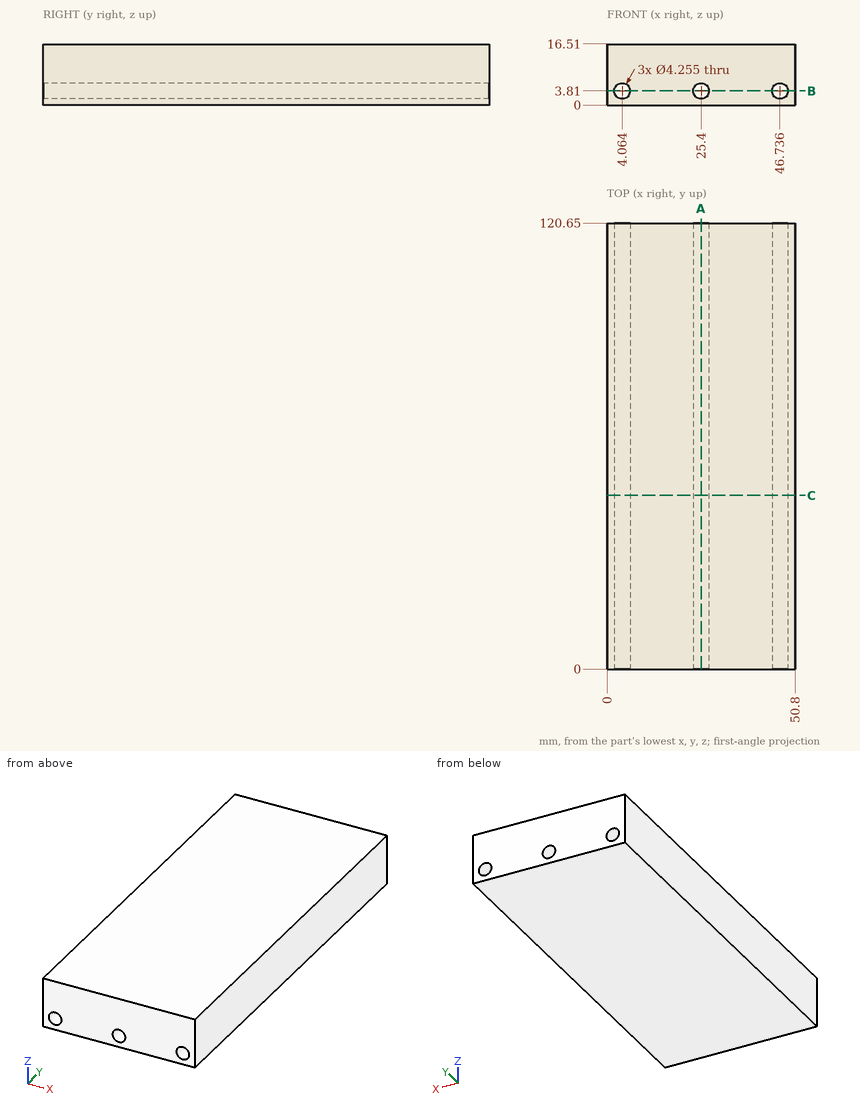
Part print with two shaded views. Sizes in mm from the minimum x, y, z corner. Give positions to 0.01 mm unless a question says otherwise; leave off trailing zeros. Order: outer loops, then holes, each group sorted by start corner. A loop starts at its lowest first (then second) coordinate and runs counter-clockwise, first axis right, second up. Notation, with made-up numbers: M 54.25,16 L 103.25,16 A20 cw 103.25,34 Z; hole C 53.5,14 d6. An arc over 180 degrees is marked long. Write item = value, one per line.
Q1. Cut at B-B, the plane z = 3.81. List the corners of the cut face in (x, y), then the cut area to 3 significant figures.
Derived:
outline = M 0,0 L 1.94,0 L 1.94,120.65 L 0,120.65 Z; M 6.19,0 L 23.27,0 L 23.27,120.65 L 6.19,120.65 Z; M 27.53,0 L 44.61,0 L 44.61,120.65 L 27.53,120.65 Z; M 48.86,0 L 50.8,0 L 50.8,120.65 L 48.86,120.65 Z
area = 4,590 mm2
Q2. Cut at A-A, the plane x = 25.4. List the corners of the cut face in (y, z), then the cut area to 3 significant figures.
Derived:
outline = M 0,0 L 120.65,0 L 120.65,1.68 L 0,1.68 Z; M 0,5.94 L 120.65,5.94 L 120.65,16.51 L 0,16.51 Z
area = 1,480 mm2
Q3. Drill centre lines: line 1 (X direction, y = 79, z = 3.81); line 2 (X direction, y = 38, z = 5.25) (1 decimal); line 3 (Z direction, x = 46, y = 9) (1 decimal). Where is each one in solid material? Low to high. Write a range as [from, to].
Derived:
line_1 = [0, 1.94], [6.19, 23.27], [27.53, 44.61], [48.86, 50.8]
line_2 = [0, 2.5], [5.6, 23.8], [27, 45.2], [48.3, 50.8]
line_3 = [0, 1.8], [5.8, 16.5]
Q4. Cut at C-C, the plane y = 47. List the corners of the cut face in (x, z) (1 decimal), then the cut area to 3 significant figures.
Derived:
outline = M 0,0 L 50.8,0 L 50.8,16.5 L 0,16.5 Z; hole C 4.1,3.8 d4.3; hole C 25.4,3.8 d4.3; hole C 46.7,3.8 d4.3
area = 796 mm2
